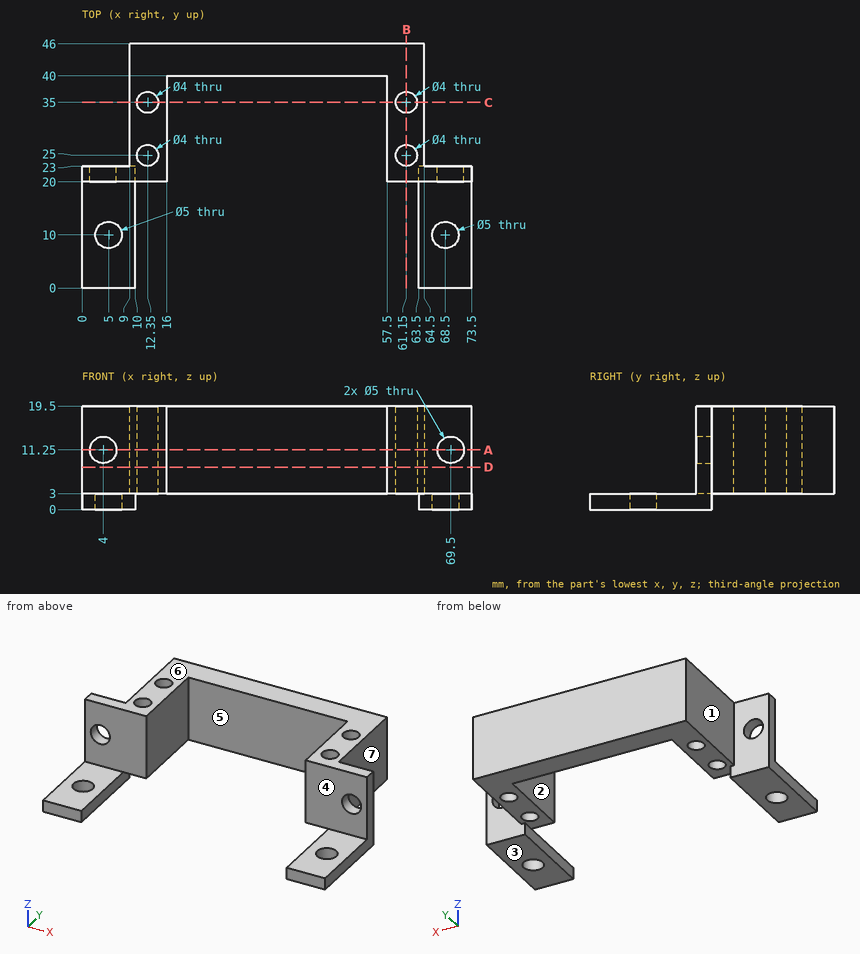
Here's the drawing with two shaded views (mm, measured from the low corner). I have some questions. A direction names the side the tool comes from. Give positions to 0.01 mm unless a question says otherwise; leave off trailing zeros. Write each loop counter-clockwise with the first axis right and the second up, starting at its lowest first coordinate (ties: lowest second). Pieces come first, ordered by that corner, then holes. Notation, with made-up numbers: (86.5, 79) - (97.5, 79) arc R24 cw to (97.5, 114) - close; hole circle Ø3 at (-25, 41.5). An arc over 180 degrees is marked (long way). One line per item, written item: value. Start each with the question number.
Item 1: I'm going to push flat-ended pins straight in: pin 1 (8 mm diameter, centred on x = 34.5, z = 8, fed in from -Y); pin 2 (4 mm diameter, centred on y = 36, z = 7, fed in from +X); pin 3 (5 mm diameter, centred on x = 71, y = 10, fed in from +Z); pin 4 (13 mm diameter, centred on x = 28.5, y = 28.5, fed in from -Z). Where does each tip first touch, or does it pass through?
Item 2: Please list where these lines run through material, in increasing order: line 1 (X direction, y = 21.05, z = 11.25); line 2 (Y direction, x = 61.15, z = 12.25); line 3 (X direction, y = 31, z = 5.25). Write a range as from..to.
Item 3: Imagine slicing it at D-D, the plane z = 8. List the corners of the cut face in (x, y) for me.
Item 4: Imagine slicing it at A-A, the plane z = 11.25. List the corners of the cut face in (x, y) for me.
Item 5: If we mould it in two halves opening along X, with no side actions, what happens to the marked faces 1, 2 and 3? For each: +X half, -X half, draft (parallel to the pull), parting line (faces both ways), or undercut.
Item 6: Imagine slicing it at B-B, the plane x = 61.15. List the corners of the cut face in (y, z) for me, and give its area (3 significant figures).
Item 7: Imagine slicing it at C-C, the plane y = 35. List the corners of the cut face in (x, z) for me.
Item 8: Which directions (+Z, -Z, +X, -X, +Y, -Y) give clear straight access to the entire face, cutting with the end or side of a thin tool? Please do the marked faces 4, 5, 6 and 7.
Geometry says:
1. pin 1: y = 40
1. pin 2: x = 64.5
1. pin 3: z = 3
1. pin 4: through
2. line 1: 0..1.5, 6.5..16, 57.5..67, 72..73.5
2. line 2: 20..23, 27..33, 37..46
2. line 3: 9..16, 57.5..64.5
3. outline: (0, 20) - (16, 20) - (16, 40) - (57.5, 40) - (57.5, 20) - (73.5, 20) - (73.5, 23) - (64.5, 23) - (64.5, 46) - (9, 46) - (9, 23) - (0, 23) - close; hole circle Ø4 at (12.35, 25); hole circle Ø4 at (12.35, 35); hole circle Ø4 at (61.15, 25); hole circle Ø4 at (61.15, 35)
4. outline: (0, 20) - (1.5, 20) - (1.5, 23) - (0, 23) - close; (6.5, 20) - (16, 20) - (16, 40) - (57.5, 40) - (57.5, 20) - (67, 20) - (67, 23) - (64.5, 23) - (64.5, 46) - (9, 46) - (9, 23) - (6.5, 23) - close; (72, 20) - (73.5, 20) - (73.5, 23) - (72, 23) - close; hole circle Ø4 at (12.35, 25); hole circle Ø4 at (12.35, 35); hole circle Ø4 at (61.15, 25); hole circle Ø4 at (61.15, 35)
5. face 1: -X half
5. face 2: undercut
5. face 3: draft
6. outline: (20, 3) - (23, 3) - (23, 19.5) - (20, 19.5) - close; (27, 3) - (33, 3) - (33, 19.5) - (27, 19.5) - close; (37, 3) - (46, 3) - (46, 19.5) - (37, 19.5) - close
6. area: 297 mm^2
7. outline: (9, 3) - (10.35, 3) - (10.35, 19.5) - (9, 19.5) - close; (14.35, 3) - (16, 3) - (16, 19.5) - (14.35, 19.5) - close; (57.5, 3) - (59.15, 3) - (59.15, 19.5) - (57.5, 19.5) - close; (63.15, 3) - (64.5, 3) - (64.5, 19.5) - (63.15, 19.5) - close
8. face 4: +Z, +X, -X, -Y
8. face 5: +Z, -Z, -Y
8. face 6: +Z, +X, -X, +Y, -Y
8. face 7: +Z, -Z, +X, +Y
